```python
from build123d import *

# Parameters (mm, degrees)
SKETCH1_W                 = 75
SKETCH1_H                 = 15
BOSS_EXTRUDE1_DEPTH       = 5
SKETCH2_W                 = 5
SKETCH2_H                 = 15
BOSS_EXTRUDE2_DEPTH       = 45
F_5_0MM_DOWEL_HOLE1_D     = 5
F_6_0MM_DOWEL_SLOT1_DEPTH = 5
BOSS_EXTRUDE3_DEPTH       = 5
BOSS_EXTRUDE7_DEPTH       = 46.8
BOSS_EXTRUDE11_DEPTH      = 8.935003
SKETCH29_W                = 15
SKETCH29_H                = 75.73500344
BOSS_EXTRUDE12_DEPTH      = 11.6
SKETCH30_W                = 75.73500344
SKETCH30_H                = 5
BOSS_EXTRUDE13_DEPTH      = 60
BOSS_EXTRUDE14_DEPTH      = 5
F_5_0MM_START             = -11.6
F_5_0MM_DOWEL_SLOT2_DEPTH = 16.6
F_5_0MM_DOWEL_SLOT3_DEPTH = 5
F_5_0MM_DOWEL_HOLE2_D     = 5


# Read off the part's stored shape, not the designer's step: Ø6.0mm Dowel Slot1, Ø5.0mm Dowel Slot2, Ø5.0mm Dowel Slot3
with BuildPart() as part:
    # Sketch1 → Boss-Extrude1 (new body)
    with BuildSketch(Plane(origin=(0, 0, 0), x_dir=(1, 0, 0), z_dir=(0, 1, 0))):
        with Locations((37.5, 7.5)):
            Rectangle(SKETCH1_W, SKETCH1_H)
    extrude(amount=BOSS_EXTRUDE1_DEPTH)

    # Sketch2 → Boss-Extrude2 (add)
    with BuildSketch(Plane(origin=(0, 5, 0), x_dir=(1, 0, 0), z_dir=(0, 1, 0))):
        with Locations((2.5, 7.5)):
            Rectangle(SKETCH2_W, SKETCH2_H)
    extrude(amount=BOSS_EXTRUDE2_DEPTH)

    # Ø5.0mm Dowel Hole1 (through all)
    with Locations(Plane.ZY):
        with Locations((-7.5, 40), (-7.5, 15)):
            Hole(F_5_0MM_DOWEL_HOLE1_D / 2)

    # Ø6.0mm Dowel Slot1 outline → Ø6.0mm Dowel Slot1 (cut)
    with BuildSketch(Plane(origin=(0, 0, 0), x_dir=(1, 0, 0), z_dir=(0, 1, 0))):
        with BuildLine():
            ThreePointArc((69.494344615, 4.96500344), (71.994344615, 7.46500344), (69.494344615, 9.96500344))
            Line((69.494344615, 9.96500344), (63.794344615, 9.96500344))
            ThreePointArc((63.794344615, 9.96500344), (61.294344615, 7.46500344), (63.794344615, 4.96500344))
            Line((63.794344615, 4.96500344), (69.494344615, 4.96500344))
        make_face()
        with BuildLine():
            ThreePointArc((56.794348468, 4.974895546), (59.294348468, 7.474895546), (56.794348468, 9.974895546))
            Line((56.794348468, 9.974895546), (51.094348468, 9.974895546))
            ThreePointArc((51.094348468, 9.974895546), (48.594348468, 7.474895546), (51.094348468, 4.974895546))
            Line((51.094348468, 4.974895546), (56.794348468, 4.974895546))
        make_face()
    extrude(amount=F_6_0MM_DOWEL_SLOT1_DEPTH, mode=Mode.SUBTRACT)

    # Sketch10 → Boss-Extrude3 (add)
    with BuildSketch(Plane.XY):
        Polygon((5, 50), (40, 5), (75, 5), (75, 0), (0, 0), (0, 50), align=None)
    extrude(amount=BOSS_EXTRUDE3_DEPTH)

    # Sketch21 → Boss-Extrude7 (add)
    with BuildSketch(Plane(origin=(0, 0, -15), x_dir=(-1, 0, 0), z_dir=(0, 0, -1))):
        Polygon((-75, 5), (-5, 5), (-5, 50), (0, 50), (0, 0), (-75, 0), align=None)
    extrude(amount=BOSS_EXTRUDE7_DEPTH)

    # Sketch22 → Boss-Extrude11 (add)
    with BuildSketch(Plane(origin=(0, 0, -61.8), x_dir=(-1, 0, 0), z_dir=(0, 0, -1))):
        Polygon((-75, 5), (-40, 5), (-5, 5), (-5, 50), (0, 50), (0, 0), (-75, 0), align=None)
    extrude(amount=BOSS_EXTRUDE11_DEPTH)

    # Sketch29 → Boss-Extrude12 (add)
    with BuildSketch(Plane.XZ):
        with Locations((7.5, -32.86750172)):
            Rectangle(SKETCH29_W, SKETCH29_H)
    extrude(amount=BOSS_EXTRUDE12_DEPTH)

    # Sketch30 → Boss-Extrude13 (add)
    with BuildSketch(Plane(origin=(15, 0, 0), x_dir=(0, 0, -1), z_dir=(1, 0, 0))):
        with Locations((32.86750172, -9.1)):
            Rectangle(SKETCH30_W, SKETCH30_H)
    extrude(amount=BOSS_EXTRUDE13_DEPTH)

    # Sketch31 → Boss-Extrude14 (add)
    with BuildSketch(Plane(origin=(0, 0, -70.73500344), x_dir=(-1, 0, 0), z_dir=(0, 0, -1))):
        Polygon((-5, 50), (-40, 5), (-5, 5), align=None)
    extrude(amount=-BOSS_EXTRUDE14_DEPTH)

    # Ø5.0mm Dowel Slot2 outline → Ø5.0mm Dowel Slot2 (cut)
    with BuildSketch(Plane(origin=(0, 0, 0), x_dir=(1, 0, 0), z_dir=(0, 1, 0)).offset(F_5_0MM_START)):
        with BuildLine():
            ThreePointArc((56.794348468, 55.774895546), (59.294348468, 58.274895546), (56.794348468, 60.774895546))
            Line((56.794348468, 60.774895546), (51.094348468, 60.774895546))
            ThreePointArc((51.094348468, 60.774895546), (48.594348468, 58.274895546), (51.094348468, 55.774895546))
            Line((51.094348468, 55.774895546), (56.794348468, 55.774895546))
        make_face()
        with BuildLine():
            ThreePointArc((69.494348468, 55.774895546), (71.994348468, 58.274895546), (69.494348468, 60.774895546))
            Line((69.494348468, 60.774895546), (63.794348468, 60.774895546))
            ThreePointArc((63.794348468, 60.774895546), (61.294348468, 58.274895546), (63.794348468, 55.774895546))
            Line((63.794348468, 55.774895546), (69.494348468, 55.774895546))
        make_face()
    extrude(amount=F_5_0MM_DOWEL_SLOT2_DEPTH, mode=Mode.SUBTRACT)

    # Ø5.0mm Dowel Slot3 outline → Ø5.0mm Dowel Slot3 (cut)
    with BuildSketch(Plane(origin=(0, 0, 0), x_dir=(1, 0, 0), z_dir=(0, 1, 0)).offset(F_5_0MM_START)):
        with BuildLine():
            Line((63.794344615, 4.96500344), (69.494344615, 4.96500344))
            ThreePointArc((69.494344615, 4.96500344), (71.994344615, 7.46500344), (69.494344615, 9.96500344))
            Line((69.494344615, 9.96500344), (63.794344615, 9.96500344))
            ThreePointArc((63.794344615, 9.96500344), (61.294344615, 7.46500344), (63.794344615, 4.96500344))
        make_face()
        with BuildLine():
            Line((51.094348468, 4.974895546), (56.794348468, 4.974895546))
            ThreePointArc((56.794348468, 4.974895546), (59.294348468, 7.474895546), (56.794348468, 9.974895546))
            Line((56.794348468, 9.974895546), (51.094348468, 9.974895546))
            ThreePointArc((51.094348468, 9.974895546), (48.594348468, 7.474895546), (51.094348468, 4.974895546))
        make_face()
    extrude(amount=F_5_0MM_DOWEL_SLOT3_DEPTH, mode=Mode.SUBTRACT)

    # Ø5.0mm Dowel Hole2 (through all)
    with Locations(Plane(origin=(5, 0, 0), x_dir=(0, 0, -1), z_dir=(1, 0, 0))):
        with Locations((58.274895546, 40), (58.274895546, 15)):
            Hole(F_5_0MM_DOWEL_HOLE2_D / 2)


solid = part.part
```
The listing builds one solid part. Answer for the finished solid, in the listing's coordinates (mm). A direction names the side the tool comes from. Coordinates: 2 decimals unless noted, no trailing zeros. Write each loop counter-clockwise with the first axis right and the second up, starting at its lowest first coordinate (ties: lowest second). Pieces come first, ordered by that corner, then holes. Notation, with made-up numbers: M 67.25,-4.75 L 113.25,-4.75 A5 cw 113.25,0.25 Z; hole C 83.5,50.25 d6. An arc over 180 degrees is marked long. Use a Markdown table: item, result. Add a question column.
1. Straight lines are drawn through the part: line 1 along Y through (x, z) = (20.5, -16); line 2 along X through (y, z) = (33, -24); line 3 along X through (y, z) = (-3, -25.5). For each, find the intervals that lie inside material, in ascending order. Write a range as [from, to].
2. Section B-B (z = -7.5) is taken. Count the separate pieces of the cut face and the enclosed holes in it, plus the area to 3 significant figures.
3. Section D-D (x = 6) is taken. Give the vertices of the cut face in (y, z) (3 decimals).
4. Section A-A (y = 40) is taken. Give the vertices of the cut face in (x, z) (3 decimals).
5. For a pull along Z with two mould halves and no side action, classify faces 4 (the flat face through (22.255, 27.815, -68.27)), 5 (the flat face through (54, 2, -9.975)) as +Z half, -Z half, draft (parallel to the pull), parting line (faces both ways), or undercut.
6. Which of the six approach directions +Z, -Z, +X, -X, +Y, -Y give full straight-line access (tool end or side, diameter ignored) to faces 1 (the flat face through (22.255, 27.815, 2.465)), 2 (the cylindrical face through (48.595, -9.135, -58.33)), 3 (the flat face through (15, 18, 0))?
7. Section C-C (z = -39.5) is taken. Give the vertices of the cut face in (x, y), plus the area to 3 significant figures.
8. Given P1, Ø4, axis at x = 48.5, z = -5, coming from the +Y side; P2, Ø2, axis at y = -5, z = -36.5, coming from the +X side; P3, Ø6.5, axis at y = 40, z = -58.27, coming from the +X side, each flat-ended and moving along its own axis, determine where each tip first touches the part or whether it passes through.
Data:
| question | item | result |
|---|---|---|
| 1 | line 1 | y = [-11.6, -6.6], [0, 5] |
| 1 | line 2 | x = [0, 5] |
| 1 | line 3 | x = [0, 15] |
| 2 | separate pieces | 7 |
| 2 | enclosed holes | 0 |
| 2 | area | 810 mm2 |
| 3 | outline | M -11.6,-70.735 L 48.714,-70.735 L 48.714,-65.735 L 5,-65.735 L 5,0 L 48.714,0 L 48.714,5 L -11.6,5 Z |
| 4 | outline | M 0,-70.735 L 12.778,-70.735 L 12.778,-65.735 L 5,-65.735 L 5,-60.775 L 0,-60.775 Z; M 0,-55.775 L 5,-55.775 L 5,-10 L 0,-10 Z; M 0,-5 L 5,-5 L 5,0 L 12.778,0 L 12.778,5 L 0,5 Z |
| 5 | face 4 | draft |
| 5 | face 5 | undercut |
| 6 | face 1 | +Z, -Z, +X, +Y |
| 6 | face 2 | +Y, -Y |
| 6 | face 3 | +X, +Y |
| 7 | outline | M 0,-11.6 L 75,-11.6 L 75,-6.6 L 15,-6.6 L 15,0 L 75,0 L 75,5 L 5,5 L 5,50 L 0,50 Z |
| 7 | area | 1,070 mm2 |
| 8 | P1 | stops at y = 5 |
| 8 | P2 | stops at x = 15 |
| 8 | P3 | stops at x = 5 |
